Design review of the part built by this model. Coordinates are the model's own, in mm. A direction names the side the tool comes from. Coordinates: 2 decimals unless noted, no trailing zeros. Write each loop counter-clockwise with the first axis right and the second up, starting at its lowest first coordinate (ties: lowest second). Pieces come first, ordered by that corner, then holes.
Q1. To check wall thickness, follow probe 1 along Y at (x, z) = (0.9, -1.75); probe 2 along Z at (x, y) = (1.6, 8); probe 3 along Y at (x, z) = (-0.2, 1.8). State the ranges of each line that lie inside material, in increasing order.
Q2. Add section A-A, the plane z = 0. Give the boundary of the cut face in (x, y).
Q3. Machinability: for faces 1 (the face through (0.3, 8, -1)), 2 (the face through (1.3, 6, 1.3)), 3 (the face through (1, 8.4, -1)), which of the approach directions +Z, -Z, +X, -X, +Y, -Y give a long, thin tool a straight path to every point of the face, cutting with its end or side? Answer none if there is none.
Q4. The part is to be moulded in two halves that separate along X. For faces 4 (the face through (-0.3, 8, -1)), 5 (the face through (-3, 7, 0)), 6 (the face through (1, 8.4, 1)), say which applies: +X half, -X half, draft (parallel to the pull), parting line (faces both ways), or undercut.
Q5. Add section C-C, the plane y = 3.5. Give the boundary of the cut face in (x, z), plus the area to 3 significant figures.
Q6. Clearance check with flat-ended pins moving along their axes: pin 1 Ø0.8 at (y, z) = (8, 1) entering from -X; pin 2 Ø0.5 at (x, y) = (1, 8) entering from +Z; pin 3 Ø0.8 at (y, z) = (8, -1) entering from +X; pin 4 Ø3 at (x, z) = (-0.5, 0) entering from +Y. State where each tip first meets the part, or that it passes through.
Q7. Add section B-B, the plane x = 0. Give the boundary of the cut face in (y, z).
Q8. Add section D-D, the plane y = 7. Give the boundary of the cut face in (x, z).
Autodesk Inventor part; units mm, degrees
ref_plane "YZ Plane" through (0, 0, 0) normal (1, 0, 0) x (0, 1, 0)
ref_plane "XZ Plane" through (0, 0, 0) normal (0, 1, 0) x (-1, 0, 0)
ref_plane "XY Plane" through (0, 0, 0) normal (0, 0, 1) x (1, 0, 0)
sketch "Sketch1" plane through (0, 0, 0) normal (0, 1, 0) x (-1, 0, 0)
  circle A0 centre (0, 0) radius 1.5
  dimension "d0" = 3
extrude "Extrusion1" add sketch "Sketch1" along normal blind 6
sketch "Sketch2" plane through (0, 6, 0) normal (0, 1, 0) x (1, 0, 0)
  circle A0 centre (0, 0) radius 1.5
  circle A1 centre (0, 0) radius 3
  dimension "d3" = 6
extrude "Extrusion2" add sketch "Sketch2" along normal blind 2.4 contours A0 | A1
fillet "Fillet4" radius 0.5 1 edges at (1.5, 0, 0)
thread "Thread2"
fillet "Fillet5" radius 1 1 edges at (-3, 8.4, 0)
sketch "Sketch5" plane through (0, 8.4, 0) normal (0, 1, 0) x (1, 0, 0)
  circle A0 centre (0, 0) radius 2
  line L0 (-0.3, 0) -> (-0.3, 1.9774)
  line L1 (0.3, 1.9774) -> (0.3, -1.9774)
  line L2 (-0.3, 1.9774) -> (-0.3, -1.9774)
  line L3 (0, 0.3) -> (-1.9774, 0.3)
  line L4 (-1.9774, 0.3) -> (1.9774, 0.3)
  line L5 (-1.9774, -0.3) -> (1.9774, -0.3)
  dimension "d32" = 0.3
  dimension "d33" = 0.3
  dimension "d35" = 0.3
  dimension "d36" = 0.3
extrude "Extrusion4" cut sketch "Sketch5" against normal blind 1 contours A0 L5 L1 L4 | L1 L4 L3 L0 A0 | L1 L5 L2 L0 L3 L4 | A0 L2 L5 L1 | L5 A0 L3 L0 L2
properties part number "M3x6"
Here are the results:
1. probe 1: y = 6 to 8.4
1. probe 2: z = -2.3 to -0.3, 0.3 to 2.3
1. probe 3: y = 6 to 7.4
2. outline: (-3, 6) - (-1.5, 6) - (-1.5, 0.5) arc R0.5 ccw to (-1, 0) - (1, 0) arc R0.5 ccw to (1.5, 0.5) - (1.5, 6) - (3, 6) - (3, 7.4) arc R1 ccw to (2, 8.4) - (2, 7.4) - (-2, 7.4) - (-2, 8.4) arc R1 ccw to (-3, 7.4) - close
3. face 1: +Y
3. face 2: -Y
3. face 3: +Z, -Z, +X, -X, +Y
4. face 4: undercut
4. face 5: parting line
4. face 6: draft
5. outline: circle Ø3 at (0, 0)
5. area: 7.07 mm2
6. pin 1: stops at x = -2.86
6. pin 2: stops at z = 2.79
6. pin 3: stops at x = 2.86
6. pin 4: stops at y = 8.4
7. outline: (0, -1) arc R0.5 ccw to (0.5, -1.5) - (6, -1.5) - (6, -3) - (7.4, -3) arc R1 ccw to (8.4, -2) - (7.4, -2) - (7.4, 2) - (8.4, 2) arc R1 ccw to (7.4, 3) - (6, 3) - (6, 1.5) - (0.5, 1.5) arc R0.5 ccw to (0, 1) - close
8. outline: circle Ø6 at (0, 0)
